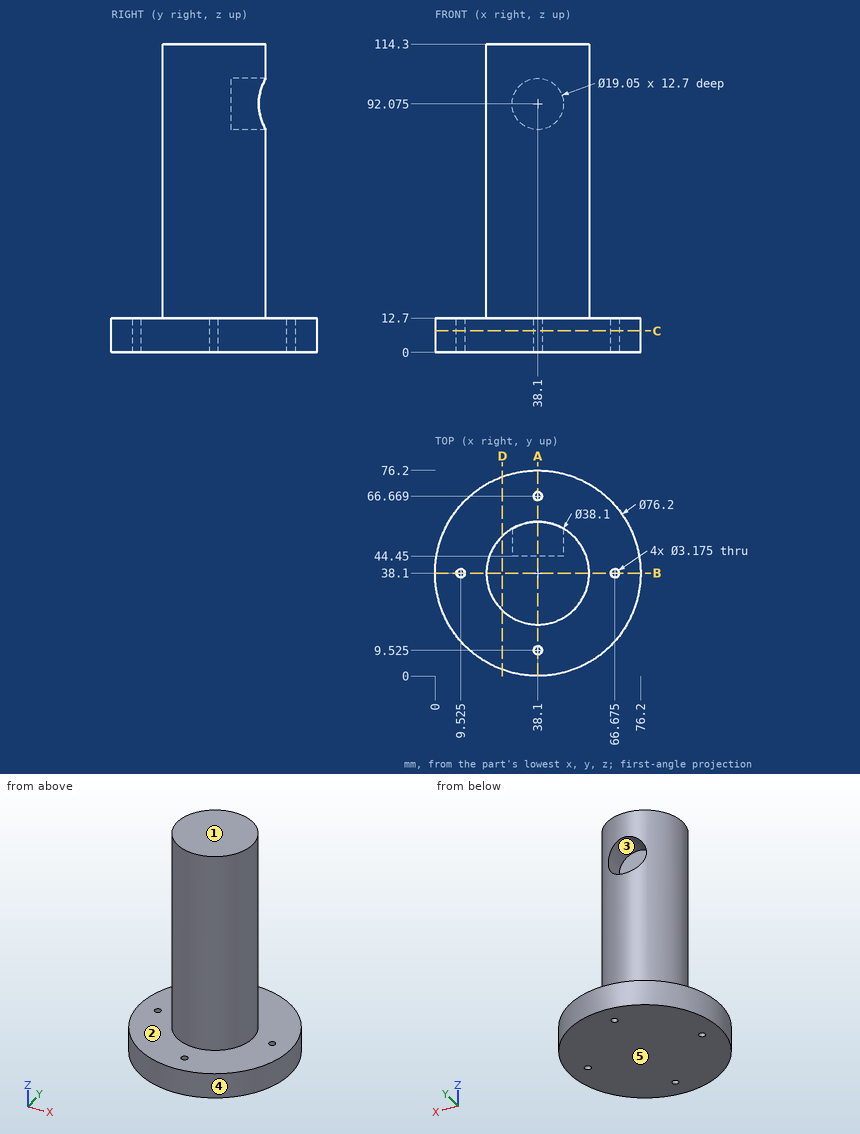
The figure shows three views and two pictorial views of one solid part (mm, origin at its lowest corner). Answer the questions. A direction names the side the tool comes from. Round coordinates to 2 decimals unless told otherwise and drop trailing zeros. Order: outer loops, then holes, each group sorted by start corner. A loop starts at its lowest first (then second) coordinate and runs counter-clockwise, first axis right, second up. Notation, with made-up numbers: M -26.75,85 L 31.25,85 A17 ccw 31.25,118 Z; hole C 86,12 d1. An arc over 180 degrees is marked long. Put each result on its own line as item: value. Start each with the question number.
Q1. Section B-B, the plane y = 38.1 is taken. Write down the section's boundary in (x, z).
Q2. Section D-D, the plane x = 25 is taken. Write down the section's boundary in (y, z), and give its area (3 significant figures).
Q3. For a pull along Z with two mould halves and no side action, classify the marked faces 3, 4 and 5 as pulls with the +Z half, pulls with the -Z half, needs draft (parallel to the pull), parting line crosses it, or undercut.
Q4. Flat-ended cylindrical pins translate along their axes: pin 1 (6 mm diameter, centred on y = 55.5, z = 45, fed in from -X); pin 2 (10 mm diameter, centred on x = 48.5, z = 28, fed in from +Y); pin 3 (10 mm diameter, centred on y = 19.5, z = 96, fed in from -X); pin 4 (4 mm diameter, centred on x = 66.675, y = 38.1, fed in from -Z). Find the tip coordinate at first contact, or state that the pin passes through.
Q5. Section C-C, the plane z = 8 is taken. Write down the section's boundary in (x, y) (1 decimal), and give its area (3 significant figures).
Q6. A tool of negligible diameter and unlimited length cuts with its end or side. For the marked faces 1 and 2, from which of +Z, -Z, +X, -X, +Y, -Y can it reach the whole face along a straight path? Write none if from no direction.
Q7. Straight lines are drawn through the part: L1, parallel to X at y = 38, z = 8; L2, parallel to Y at x = 38.1, z = 7.75; L3, parallel to Z at x = 38.1, y = 50. For each, find the intervals that lie inside material, in ascending order. Write a range as [from, to].
Q8. Section A-A, the plane x = 38.1 is taken. Write down the section's boundary in (y, z), and give its area (3 significant figures).
Findings below:
1. outline: M 0,0 L 7.94,0 L 7.94,12.7 L 0,12.7 Z; M 11.11,0 L 65.09,0 L 65.09,12.7 L 57.15,12.7 L 57.15,114.3 L 19.05,114.3 L 19.05,12.7 L 11.11,12.7 Z; M 68.26,0 L 76.2,0 L 76.2,12.7 L 68.26,12.7 Z
2. outline: M 2.32,0 L 73.88,0 L 73.88,12.7 L 51.93,12.7 L 51.93,114.3 L 24.27,114.3 L 24.27,12.7 L 2.32,12.7 Z
2. area: 3,720 mm^2
3. face 3: undercut
3. face 4: needs draft
3. face 5: pulls with the -Z half
4. pin 1: stops at x = 25.63
4. pin 2: stops at y = 56.37
4. pin 3: stops at x = 24.76
4. pin 4: stops at z = 0
5. outline: C 38.1,38.1 d76.2; hole C 9.5,38.1 d3.2; hole C 38.1,9.5 d3.2; hole C 38.1,66.7 d3.2; hole C 66.7,38.1 d3.2
5. area: 4,530 mm^2
6. face 1: +Z, +X, -X, +Y, -Y
6. face 2: +Z
7. L1: x = [0, 7.94], [11.11, 65.09], [68.26, 76.2]
7. L2: y = [0, 7.94], [11.11, 65.08], [68.26, 76.2]
7. L3: z = [0, 82.55], [101.6, 114.3]
8. outline: M 0,0 L 7.94,0 L 7.94,12.7 L 0,12.7 Z; M 11.11,0 L 65.08,0 L 65.08,12.7 L 57.15,12.7 L 57.15,82.55 L 44.45,82.55 L 44.45,101.6 L 57.15,101.6 L 57.15,114.3 L 19.05,114.3 L 19.05,12.7 L 11.11,12.7 Z; M 68.26,0 L 76.2,0 L 76.2,12.7 L 68.26,12.7 Z
8. area: 4,520 mm^2
